Read the model definition and answer for the solid it produces. Units are mm, in the model's axes. A direction names the side the tool comes from. Coordinates: 2 decimals unless noted, no trailing zeros. Loops run counter-clockwise (first coordinate to the right, second up) from the corner with the lowest first, then second, coordinate; pieces in that order, holes last. Notation, with made-up numbers: (-9.5, -2.75) - (42.5, -2.75) arc R27 cw to (42.5, 25.25) - close; hole circle Ø2 at (54, 23). An arc over 180 degrees is marked (long way). Use one line per item in the form item = value. Start each with the question number.
1) The mould has two halves that part along Z. Classify faces 5 (the face through (5, -4, 18)), 6 (the face through (-3.4, -2.2, 0)), 7 (the face through (-0.594, -4.24, 22.932)): released by +Z, released by -Z, zero draft, split by the parting line, or undercut.
2) A cutting plane is placed at A-A (z = 21.5). Give the vertices of the cut face in (x, y), and give its area (4 significant figures).
3) Which of the six approach directions +Z, -Z, +X, -X, +Y, -Y give full straight-line access (tool end or side, diameter ignored) to faces 1 (the face through (3, -3, 25)), 2 (the face through (4.27, -2.75, 17.97)), 3 (the face through (-3.494, 0.199, 5.423)), 4 (the face through (4, -2.5, 6))?
4) Consider line 1 (X direction, y = -4.7, z = 14.5); line 2 (Z direction, x = -3.5, y = -1.75); line 3 (X direction, y = 0, z = 6). Determine where each line is inside the solid, lowest interval first.
5) Each of these flat-tipped pins is pushed along its axis until it touches: P1, Ø5, axis at x = 2, z = 18.5, coming from the +Y side; P2, Ø2, axis at x = 3.5, z = 28, coming from the +Y side; P3, Ø1.5, axis at x = 1.5, z = 24.5, coming from the +Y side. Where does it stop, or does it pass through?
6) A cutting plane is placed at B-B (y = -4). Give the vertices of the cut face in (x, z).
7) A cutting plane is placed at C-C (y = 1.25). Give the vertices of the cut face in (x, z), and give its area (3 significant figures).
8) A cutting plane is placed at D-D (z = 3.5). Give the vertices of the cut face in (x, y).
from build123d import *

# Parameters (mm, degrees)
RESSALTO_EXTRUS_O1_DEPTH = 11
ESBO_O2_W                = 10
ESBO_O2_H                = 1.5
RESSALTO_EXTRUS_O2_DEPTH = 7
RESSALTO_EXTRUS_O3_DEPTH = 2
ESBO_O4_R                = 1.55
CORTE_EXTRUS_O1_DEPTH    = 2
CORTE_EXTRUS_O2_DEPTH    = 37.687872656


with BuildPart() as part:
    # Esboço1 → Ressalto-extrusão1 (new body)
    with BuildSketch(Plane.XY):
        with BuildLine():
            Line((-5, -5), (0, -5))
            ThreePointArc((0, -5), (-3.535533906, -3.535533906), (-5, 0))
            Line((-5, 0), (-5, -5))
        make_face()
        with BuildLine():
            Line((5, -5), (5, 0))
            ThreePointArc((5, 0), (3.535533906, -3.535533906), (0, -5))
            Line((0, -5), (5, -5))
        make_face()
        with BuildLine():
            ThreePointArc((-3.5, 0), (0, 3.5), (3.5, 0))
            Line((3.5, 0), (5, 0))
            ThreePointArc((5, 0), (3.535533906, 3.535533905), (1e-09, 5))
            ThreePointArc((1e-09, 5), (-3.535533905, 3.535533906), (-5, 0))
            Line((-5, 0), (-3.5, 0))
        make_face()
        with BuildLine():
            Line((5, 0), (3.5, 0))
            ThreePointArc((3.5, 0), (0, -3.5), (-3.5, 0))
            Line((-3.5, 0), (-5, 0))
            ThreePointArc((-5, 0), (-3.535533906, -3.535533906), (0, -5))
            ThreePointArc((0, -5), (3.535533906, -3.535533906), (5, 0))
        make_face()
    ressalto_extrus_o1 = extrude(amount=RESSALTO_EXTRUS_O1_DEPTH)

    # Esboço2 → Ressalto-extrusão2 (add)
    with BuildSketch(Plane.XY.offset(11)):
        with Locations((0, -4.25)):
            Rectangle(ESBO_O2_W, ESBO_O2_H)
    ressalto_extrus_o2 = extrude(amount=RESSALTO_EXTRUS_O2_DEPTH)

    # Esboço3 → Ressalto-extrusão3 (add)
    with BuildSketch(Plane.XY.offset(18)):
        with BuildLine():
            Line((3.5, -3.5), (5, -3.5))
            ThreePointArc((5, -3.5), (4.25, -2.75), (3.5, -3.5))
        make_face()
        with BuildLine():
            Line((-5, -3.5), (-3.5, -3.5))
            ThreePointArc((-3.5, -3.5), (-4.25, -2.75), (-5, -3.5))
        make_face()
    ressalto_extrus_o3 = extrude(amount=-RESSALTO_EXTRUS_O3_DEPTH)

    # Espelhar1: Ressalto-extrusão1, Ressalto-extrusão2, Ressalto-extrusão3 across plane
    add(ressalto_extrus_o1.mirror(Plane(origin=(0, 0, 18), x_dir=(1, 0, 0), z_dir=(0, 0, -1))))
    add(ressalto_extrus_o2.mirror(Plane(origin=(0, 0, 18), x_dir=(1, 0, 0), z_dir=(0, 0, -1))))
    add(ressalto_extrus_o3.mirror(Plane(origin=(0, 0, 18), x_dir=(1, 0, 0), z_dir=(0, 0, -1))))

    # Esboço4 → Corte-extrusão1 (cut)
    with BuildSketch(Plane(origin=(0, -3.5, 0), x_dir=(1, 0, 0), z_dir=(0, 1, 0))):
        with Locations(Location((0, -14.5, 0), (0, 0, 270))):
            Circle(ESBO_O4_R)
        with Locations(Location((0, -21.5, 0), (0, 0, 270))):
            Circle(ESBO_O4_R)
    extrude(amount=-CORTE_EXTRUS_O1_DEPTH, mode=Mode.SUBTRACT)

    # Esboço5 → Corte-extrusão2 (cut, through all)
    with BuildSketch(Plane.XY.offset(36)):
        with BuildLine():
            Line((2.449489743, -2.5), (5, -2.5))
            Line((5, -2.5), (5, 0))
            ThreePointArc((5, 0), (4.766431527, 1.510341187), (4.087547799, 2.87957514))
            Line((4.087547799, 2.87957514), (2.861283459, 2.015702598))
            ThreePointArc((2.861283459, 2.015702598), (3.336502069, 1.057238831), (3.5, 0))
            ThreePointArc((3.5, 0), (3.226702194, -1.355873501), (2.449489743, -2.5))
        make_face()
    extrude(amount=-CORTE_EXTRUS_O2_DEPTH, mode=Mode.SUBTRACT)


solid = part.part
Found:
q1.face_5 = zero draft
q1.face_6 = released by -Z
q1.face_7 = undercut
q2.outline = (-5, -5) - (-1.55, -5) - (-1.55, -3.5) - (-5, -3.5) - close; (1.55, -5) - (5, -5) - (5, -3.5) - (1.55, -3.5) - close
q2.area = 10.35 mm^2
q3.face_1 = +X, -X, +Y
q3.face_2 = +Y
q3.face_3 = +Z, -Z
q3.face_4 = +Z, -Z, +X
q4.line_1 = -5 to -1.55, 1.55 to 5
q4.line_2 = 0 to 11, 25 to 36
q4.line_3 = -5 to -3.5
q5.P1 = -2.75
q5.P2 = 4.33
q5.P3 = 4.91
q6.outline = (-5, 0) - (5, 0) - (5, 36) - (-5, 36) - close; hole circle Ø3.1 at (0, 14.5); hole circle Ø3.1 at (0, 21.5)
q7.outline = (-4.84, 0) - (-3.27, 0) - (-3.27, 11) - (-4.84, 11) - close; (-4.84, 25) - (-3.27, 25) - (-3.27, 36) - (-4.84, 36) - close
q7.area = 34.6 mm^2
q8.outline = (-5, -5) - (5, -5) - (5, -2.5) - (2.45, -2.5) arc R3.5 cw (long way) to (2.86, 2.02) - (4.09, 2.88) arc R5 ccw to (-5, 0) - close
